from build123d import *

# Parameters (mm, degrees)
CHANFREIN1_SIZE         = 0.5
ENL_V_MAT_EXTRU_1_DEPTH = 1.2


with BuildPart() as part:
    # Esquisse1 → Révolution1 (revolve)
    with BuildSketch(Plane.XY):
        Polygon((0, 0), (0, 3), (0.2, 3), (1.7, 1.5), (10, 1.5), (10, 0), align=None)
    revolve(axis=Axis((10, 0, 0), (-1, 0, 0)))

    # Chanfrein1
    chanfrein1_edges = [part.edges().sort_by_distance(p)[0] for p in [
        (10, -1.5, 0),
    ]]
    chamfer(chanfrein1_edges, length=CHANFREIN1_SIZE)

    # Esquisse2 → Enlèv. mat.-Extru.1 (cut)
    with BuildSketch(Plane.ZY):
        Polygon((0, 1.154700538), (-1, 0.577350269), (-1, -0.577350269), (0, -1.154700538), (1, -0.577350269), (1, 0.577350269), align=None)
    extrude(amount=-ENL_V_MAT_EXTRU_1_DEPTH, mode=Mode.SUBTRACT)


solid = part.part
Design review of the part built by this model. Coordinates are the model's own, in mm. A direction names the side the tool comes from. Round coordinates to 2 decimals unless told otherwise and drop trailing zeros. Write each loop counter-clockwise with the first axis right and the second up, starting at its lowest first coordinate (ties: lowest second). Pieces come first, ordered by that corner, then holes. Notation, with made-up numbers: (35, 13.25) - (56, 13.25) arc R13 cw to (56, 26.25) - close; hole circle Ø5 at (58, 67.25). An arc over 180 degrees is marked (long way). Use a Markdown table: item, result. Add a question column.
1. Wall thickness on probe 1 along X at (y, z) = (0.8, 0.5); probe 2 along Y at (x, z) = (6.25, -0.1); probe 3 along X at (y, z) = (-0.4, -2.2): over which ranges is each line inside the solid? List them lowest first.
2. Clearance check with flat-ended pins moving along their axes: pin 1 (1 mm diameter, centred on y = -1.5, z = 1.5, fed in from +X); pin 2 (1.6 mm diameter, centred on y = 0, z = 0, fed in from -X); pin 3 (2 mm diameter, centred on x = 2, y = 0, fed in from -Z). State where each tip first meets the part, or that it passes through.
3. Mouldability with a two-part tool opening along Y and no side actions: class faces 1 (the face through (0, 0, 1.3)), 2 (the face through (5.65, -1.5, -0.07)), 3 (the face through (0.59, 0.86, 0.51)) as +Y half, -Y half, draft (parallel to the pull), parting line (faces both ways), or undercut.
4. We need section A-A (y = 0). State the section outline as (x, z) points.
5. We need section B-B (x = 2.75). State the section outline as (y, z) points.
6. For faces 4 (the face through (1, 0, 1)), 5 (the face through (10, 0, 0)), list the 3-axis set-ups (+Z, -Z, +X, -X, +Y, -Y) from which the entire face can be reached by the end or side of a thin tool; tool diameter is ignored.
Output:
| question | item | result |
|---|---|---|
| 1 | probe 1 | x = 1.2 to 10 |
| 1 | probe 2 | y = -1.5 to 1.5 |
| 1 | probe 3 | x = 0 to 0.96 |
| 2 | pin 1 | stops at x = 1.58 |
| 2 | pin 2 | stops at x = 1.2 |
| 2 | pin 3 | stops at z = -2.2 |
| 3 | face 1 | draft |
| 3 | face 2 | parting line |
| 3 | face 3 | undercut |
| 4 | outline | (0, -3) - (0.2, -3) - (1.7, -1.5) - (9.5, -1.5) - (10, -1) - (10, 1) - (9.5, 1.5) - (1.7, 1.5) - (0.2, 3) - (0, 3) - (0, 1) - (1.2, 1) - (1.2, -1) - (0, -1) - close |
| 5 | outline | circle Ø3 at (0, 0) |
| 6 | face 4 | -X |
| 6 | face 5 | +Z, -Z, +X, +Y, -Y |
